Autodesk Inventor part; units mm, degrees
ref_plane "YZ Plane" through (0, 0, 0) normal (1, 0, 0) x (0, 1, 0)
ref_plane "XZ Plane" through (0, 0, 0) normal (0, 1, 0) x (-1, 0, 0)
ref_plane "XY Plane" through (0, 0, 0) normal (0, 0, 1) x (1, 0, 0)
sketch "Sketch1" plane through (0, 0, 0) normal (0, 0, 1) x (1, 0, 0)
  circle A0 centre (0, 0) radius 9.6012
  circle A1 centre (-16.256, 0) radius 4.7625
  circle A2 centre (16.256, 0) radius 4.7625
  line L0 (7.9375, 14.224) -> (-7.9375, 14.224)
  line L1 (-7.9375, 14.224) -> (-27.5622, 4.2576)
  circle A3 centre (-25.4, 0) radius 2.5527
  arc A4 (-27.5622, 4.2576) -> (-27.5622, -4.2576) centre (-25.4, 0) ccw
  line L2 (-27.5622, -4.2576) -> (-7.9375, -14.224)
  line L3 (-7.9375, -14.224) -> (7.9375, -14.224)
  circle A5 centre (25.4, 0) radius 2.5527
  arc A6 (27.5622, -4.2576) -> (27.5622, 4.2576) centre (25.4, 0) ccw
  line L4 (7.9375, 14.224) -> (27.5622, 4.2576)
  line L5 (27.5622, -4.2576) -> (7.9375, -14.224)
  point P0 (0, 14.224)
  point P1 (0, -14.224)
  dimension "d0" = 19.2024
  dimension "d1" = 9.525
  dimension "d2" = 16.256
  dimension "d3" = 16.256
  dimension "d4" = 15.875
  dimension "d5" = 5.1054
  dimension "d6" = 25.4
  dimension "d7" = 4.7752
  dimension "d8" = 28.448
  dimension "d9" = 5.1054
  dimension "d10" = 25.4
  dimension "d11" = 4.7752
  dimension "d12" = 14.224
extrude "Extrusion1" add sketch "Sketch1" along normal blind 3.175
properties part number "CIM Spacer" material "Aluminum 6061"
The listing builds one solid part. Answer for the finished solid, in the listing's coordinates (mm). Give positions to 0.01 mm unless a question says otherwise; leave off trailing zeros. Order: outer loops, then holes, each group sorted by start corner. A loop starts at its lowest first (then second) coordinate and runs counter-clockwise, first axis right, second up. Notation, with made-up numbers: M 87.5,-32 L 134.5,-32 A25 cw 134.5,-5 Z; hole C 46.25,58.25 d9. An arc over 180 degrees is marked long. Put each result on its own line as item: value. Start each with the question number.
Item 1: Find the intervals of material crossed by line 1 along X through (y, z) = (-0.5, 1.3); line 2 along Y through (x, z) = (-25.4, 0.7); line 3 along Y through (x, z) = (3, 1.55), in increasing order.
Item 2: The part is cut by section D-D, the plane y = 8.75. Determine the outline of the cut face in (x, z) (3 decimals).
Item 3: For a pull along Y with two mould halves and no side action, classify faces 1 (the face through (-17.89, -9.17, 1.57)), 2 (the face through (0, 14.224, 2)), 3 (the face through (-27.95, -0.11, 1.57)) as +Y half, -Y half, draft (parallel to the pull), parting line (faces both ways), or undercut.
Item 4: A flat-ended cylindrical pin translates along its axis: P1, Ø1.5, axis at x = -17.5, z = 2.5, coming from the -Y side. Find the tip coordinate at first contact, or state that the pin passes through.
Item 5: The part is cut by section B-B, the plane z = 1.9. Determine the outline of the cut face in (x, y) (1 decimal).
Item 6: The part is cut by section A-A, the plane x = 0. Determine the outline of the cut face in (y, z) (3 decimals).
Item 7: The part is cut by section C-C, the plane y = 0. Determine the outline of the cut face in (x, z) (1 decimal).
Answer key:
1. line 1: x = -30.15 to -27.9, -22.9 to -20.99, -11.52 to -9.59, 9.59 to 11.52, 20.99 to 22.9, 27.9 to 30.15
1. line 2: y = -5.36 to -2.55, 2.55 to 5.36
1. line 3: y = -14.22 to -9.12, 9.12 to 14.22
2. outline: M -18.716,0 L -3.952,0 L -3.952,3.175 L -18.716,3.175 Z; M 3.952,0 L 18.716,0 L 18.716,3.175 L 3.952,3.175 Z
3. face 1: -Y half
3. face 2: +Y half
3. face 3: undercut
4. P1: stops at y = -9.75
5. outline: M -27.6,-4.3 L -7.9,-14.2 L 7.9,-14.2 L 27.6,-4.3 A4.8 ccw 27.6,4.3 L 7.9,14.2 L -7.9,14.2 L -27.6,4.3 A4.8 ccw Z; hole C -25.4,0 d5.1; hole C -16.3,0 d9.5; hole C 0,0 d19.2; hole C 16.3,0 d9.5; hole C 25.4,0 d5.1
6. outline: M -14.224,0 L -9.601,0 L -9.601,3.175 L -14.224,3.175 Z; M 9.601,0 L 14.224,0 L 14.224,3.175 L 9.601,3.175 Z
7. outline: M -30.2,0 L -28,0 L -28,3.2 L -30.2,3.2 Z; M -22.8,0 L -21,0 L -21,3.2 L -22.8,3.2 Z; M -11.5,0 L -9.6,0 L -9.6,3.2 L -11.5,3.2 Z; M 9.6,0 L 11.5,0 L 11.5,3.2 L 9.6,3.2 Z; M 21,0 L 22.8,0 L 22.8,3.2 L 21,3.2 Z; M 28,0 L 30.2,0 L 30.2,3.2 L 28,3.2 Z
